from build123d import *

# Parameters (mm, degrees)
BOSS_EXTRUDE1_DEPTH = 3
SKETCH3_W           = 3.3
SKETCH3_H           = 10
CUT_EXTRUDE1_DEPTH  = 4
FILLET1_R           = 3


with BuildPart() as part:
    # Sketch1 → Boss-Extrude1 (new body)
    with BuildSketch(Plane.XY):
        with BuildLine():
            Line((86.496300823, -131.179339344), (85.797718449, -131.179339344))
            ThreePointArc((85.797718449, -131.179339344), (84.643346916, -130.896866427), (83.749838339, -130.113280435))
            Line((83.749838339, -130.113280435), (3.007715481, -14.801578616))
            ThreePointArc((3.007715481, -14.801578616), (0.208070871, -13.85122733), (-1.54016463, -16.235519707))
            Line((-1.54016463, -16.235519707), (-1.54016463, -151.684305639))
            ThreePointArc((-1.54016463, -151.684305639), (1.388767558, -158.75537345), (8.45983537, -161.684305639))
            Line((8.45983537, -161.684305639), (91.483543137, -161.684305639))
            ThreePointArc((91.483543137, -161.684305639), (98.554610949, -158.75537345), (101.483543137, -151.684305639))
            Line((101.483543137, -151.684305639), (101.483543137, -124.184305639))
            ThreePointArc((101.483543137, -124.184305639), (100.75131009, -122.416538686), (98.983543137, -121.684305639))
            Line((98.983543137, -121.684305639), (98.629733048, -121.684305639))
            ThreePointArc((98.629733048, -121.684305639), (97.08903242, -122.215488335), (96.203046603, -123.58331238))
            ThreePointArc((96.203046603, -123.58331238), (92.659103337, -129.054608557), (86.496300823, -131.179339344))
        make_face()
    extrude(amount=BOSS_EXTRUDE1_DEPTH)

    # Sketch3 → Cut-Extrude1 (cut, through all)
    with BuildSketch(Plane(origin=(0, 0, 0), x_dir=(-1, 0, 0), z_dir=(0, 0, -1))):
        with Locations((-49.971689254, -156.684305639)):
            Rectangle(SKETCH3_W, SKETCH3_H)
        with Locations((-21.671689254, -156.684305639)):
            Rectangle(SKETCH3_W, SKETCH3_H)
        with Locations((-78.271689254, -156.684305639)):
            Rectangle(SKETCH3_W, SKETCH3_H)
    extrude(amount=-CUT_EXTRUDE1_DEPTH, mode=Mode.SUBTRACT)

    # Fillet1
    fillet1_edges = [part.edges().sort_by_distance(p)[0] for p in [
        (23.321689254, -161.684305639, 1.5),
        (20.021689254, -161.684305639, 1.5),
        (76.621689254, -161.684305639, 1.5),
        (79.921689254, -161.684305639, 1.5),
        (48.321689254, -161.684305639, 1.5),
        (51.621689254, -161.684305639, 1.5),
    ]]
    fillet(fillet1_edges, radius=FILLET1_R)


solid = part.part
Part model, mm, in its own coordinate system. A direction names the side the tool comes from. Round coordinates to 2 decimals unless told otherwise and drop trailing zeros. Write each loop counter-clockwise with the first axis right and the second up, starting at its lowest first coordinate (ties: lowest second). Pieces come first, ordered by that corner, then holes. Notation, with made-up numbers: (84.25, 27) - (94.25, 27) arc R17 ccw to (94.25, 38) - close; hole circle Ø5 at (56, -22). An arc over 180 degrees is marked (long way). Use CSV: the item, a comma, the result in double quotes.
Item 1: Pull direction X, two halves, no side cores. Call faces 1 (the cylindrical face through (80.824, -160.829, 1.521)), 2 (the flat face through (-1.54, -83, 1)), 3 (the cylindrical face through (98.48, -158.83, 1.48)): pulls with the +X half, pulls with the -X half, needs draft (parallel to the pull), parting line crosses it, or undercut.
Results list:
face 1,"undercut"
face 2,"pulls with the -X half"
face 3,"pulls with the +X half"
Item 2: Slice it at B-B, the plane y = -33.5. Write the cut outline in (x, z), then the cut area to 3 significant figures.
Results list:
outline,"(-1.54, 0) - (16.1, 0) - (16.1, 3) - (-1.54, 3) - close"
area,"52.9 mm²"
Item 3: Slice it at C-C, the plane x = 66. Write the cut outline in (y, z).
Results list:
outline,"(-161.68, 0) - (-104.76, 0) - (-104.76, 3) - (-161.68, 3) - close"
Item 4: Tool access for faces 4 (the cylindrical face through (1.311, -158.677, 1.479)), 5 (the flat face through (79.922, -155, 1)): list every direction of +Z, -Z, +X, -X, +Y, -Y with a clear straight run to the whole face (end or side of a thin tool).
Results list:
face 4,"+Z, -Z, -X, -Y"
face 5,"+Z, -Z, -Y"
Item 5: Flat gauge pins, fed straight in: P1, Ø1.5, axis at y = -155.5, z = 1.5, coming from the -X side; P2, Ø1.5, axis at y = -155, z = 1, coming from the -X side; P3, Ø0.9, axis at y = -155.5, z = 1.5, coming from the +X side; P4, Ø5, axis at x = 72.5, y = -118.5, coming from the -Z side. Where does each tip first touch, or does it go through?
Results list:
P1,"stops at x = -1.06"
P2,"stops at x = -1.21"
P3,"stops at x = 100.9"
P4,"stops at z = 0"
Item 6: Wall check: L1, parallel to X at y = -154.5, z = 2.8; L2, parallel to X at y = -33, z = 0.4; L3, parallel to Y at x = 66, z = 2.6. Give the ranges that are in metal, low to high.
Results list:
L1,"x = -1.14 to 20.02, 23.32 to 48.32, 51.62 to 76.62, 79.92 to 101.08"
L2,"x = -1.54 to 15.75"
L3,"y = -161.68 to -104.76"
